Build history of the part. All positions in model axes, mm. A direction names the side the tool comes from. Round coordinates to 2 decimals unless told otherwise and drop trailing zeros. Order: outer loops, then holes, each group sorted by start corner. A loop starts at its lowest first (then second) coordinate and runs counter-clockwise, first axis right, second up. Notation, with made-up numbers: (49, 71.25) -> (100, 71.25) arc R5 ccw to (100, 78.25) -> close; hole circle Ø10 at (69, 1). An arc over 180 degrees is marked (long way). Write item = value, one per line.
from build123d import *

# Parameters (mm, degrees)
FILLET_1_R      = 0.3
FILLET_2_R      = 0.3
SKETCH_2_W      = 0.5
SKETCH_2_H      = 0.4
EXTRUDE_1_DEPTH = 5
SKETCH_3_W      = 0.7
SKETCH_3_H      = 0.6
EXTRUDE_2_DEPTH = 1.5
SKETCH_5_W      = 0.5
SKETCH_5_H      = 0.4
EXTRUDE_3_DEPTH = 9.5
SWEEP_START     = -1.52
SWEEP_2_DEPTH   = 0.5
SKETCH_7_262_W  = 0.5
SKETCH_7_262_H  = 0.4


# Read off the part's stored shape, not the designer's step: По траектории2
with BuildPart() as part:
    # Эскиз1 → Повернуть2 (revolve)
    with BuildSketch(Plane(origin=(0, 0, 0), x_dir=(0, 0, -1), z_dir=(1, 0, 0))):
        with BuildLine():
            Line((0, 0), (-2, 0))
            Line((-2, 0), (-2, 1))
            Line((-2, 1), (-1.5, 1))
            Line((-1.5, 1), (-1.5, 4))
            ThreePointArc((-1.5, 4), (-1.07971355, 5.07971355), (0, 5.5))
            Line((0, 5.5), (0, 0))
        make_face()
    revolve(axis=Axis((0, 5.5, 0), (0, -1, 0)))

    # Скругление1
    fillet_1_edges = [part.edges().sort_by_distance(p)[0] for p in [
        (0, 1, -2),
    ]]
    fillet(fillet_1_edges, radius=FILLET_1_R)

    # Скругление2
    fillet_2_edges = [part.edges().sort_by_distance(p)[0] for p in [
        (0, 1, -1.5),
    ]]
    fillet(fillet_2_edges, radius=FILLET_2_R)

    # Эскиз2 → Вытянуть1 (add)
    with BuildSketch(Plane.XZ):
        with Locations((-1.27, 0)):
            Rectangle(SKETCH_2_W, SKETCH_2_H)
        with Locations((1.27, 0)):
            Rectangle(SKETCH_2_W, SKETCH_2_H)
    extrude(amount=EXTRUDE_1_DEPTH)

    # Эскиз3 → Вытянуть2 (add)
    with BuildSketch(Plane.XZ.offset(5)):
        with Locations((-1.27, 0)):
            Rectangle(SKETCH_3_W, SKETCH_3_H)
        with Locations((1.27, 0)):
            Rectangle(SKETCH_3_W, SKETCH_3_H)
    extrude(amount=EXTRUDE_2_DEPTH)

    # Эскиз5 → Вытянуть3 (add)
    with BuildSketch(Plane.XZ.offset(6.5)):
        with Locations((-1.27, 0)):
            Rectangle(SKETCH_5_W, SKETCH_5_H)
        with Locations((1.27, 0)):
            Rectangle(SKETCH_5_W, SKETCH_5_H)
    extrude(amount=EXTRUDE_3_DEPTH)

    # По траектории2 outline → По траектории2 (add)
    with BuildSketch(Plane.YZ.offset(SWEEP_START)):
        with BuildLine():
            Line((-17.2, -3), (-16.8, -3))
            Line((-16.8, -3), (-16.8, -0.5))
            ThreePointArc((-16.8, -0.5), (-16.712132034, -0.287867966), (-16.5, -0.2))
            Line((-16.5, -0.2), (-16, -0.2))
            Line((-16, -0.2), (-16, 0.2))
            Line((-16, 0.2), (-16.5, 0.2))
            ThreePointArc((-16.5, 0.2), (-16.994974747, -0.005025253), (-17.2, -0.5))
            Line((-17.2, -0.5), (-17.2, -3))
        make_face()
    extrude(amount=SWEEP_2_DEPTH)

    # По траектории11: sweep along a curve in space
    with BuildLine() as sweep_11_path:
        Line((-1.27, -16, 0), (-1.27, -16.5, 0))
        ThreePointArc((-1.27, -16.5, 0), (-1.27, -16.853553391, -0.146446609), (-1.27, -17, -0.5))
        Line((-1.27, -17, -0.5), (-1.27, -17, -3))
    # Эскиз7<262> → По траектории11 (sweep)
    with BuildSketch(Plane.XZ.offset(16)):
        with Locations((-1.27, 0)):
            Rectangle(SKETCH_7_262_W, SKETCH_7_262_H)
        with Locations((1.27, 0)):
            Rectangle(SKETCH_7_262_W, SKETCH_7_262_H)
    sweep(path=sweep_11_path.line)


solid = part.part
Q1. Cut at A-A, the plane y = -6. List the corners of the cut face in (x, z).
Check values:
outline = (-1.62, -0.3) -> (-0.92, -0.3) -> (-0.92, 0.3) -> (-1.62, 0.3) -> close; (0.92, -0.3) -> (1.62, -0.3) -> (1.62, 0.3) -> (0.92, 0.3) -> close
Q2. Probe probe 1 along Y at (x, z) = (1.05, -2.15); probe 2 along Y at (x, z) = (0.95, -1.65); probe 3 along Z at (x, y) = (-1.2, -7). List the from-to ranges inside material, lowest first.
Check values:
probe_1 = -17.2 to -16.8
probe_2 = 0 to 0.92
probe_3 = -0.2 to 0.2
Q3. Cut at D-D, the plane y = 2. List the corners of the cut face in (x, z), and give its area (3 significant figures).
Check values:
outline = circle Ø3 at (0, 0)
area = 7.07 mm²
Q4. Cut at B-B, the plane y = -12.25. List the corners of the cut face in (x, z).
Check values:
outline = (-1.52, -0.2) -> (-1.02, -0.2) -> (-1.02, 0.2) -> (-1.52, 0.2) -> close; (1.02, -0.2) -> (1.52, -0.2) -> (1.52, 0.2) -> (1.02, 0.2) -> close
Q5. Flat gauge pins, fed straight in: pin 1 (0.8 mm diameter, centred on x = -1.5, y = -6, fed in from +Z); pin 2 (0.7 mm diameter, centred on x = 1.5, z = 0, fed in from +Y); pin 3 (1 mm diameter, centred on y = -4.5, z = -0.5, fed in from +X). Where does each tip first touch, or does it go through?
Check values:
pin_1 = 0.3
pin_2 = 5
pin_3 = 1.52
Q6. Which spindle directions (+Z, -Z, +X, -X, +Y, -Y) get a long thin tool onto all of the face, cutting with end or side? Do faces 1 (the face through (-1.02, -13, 0)), 2 (the face through (1.952, 0.355, -0.434)), 3 (the face through (1.52, -13, 0)). Say none if no direction does.
Check values:
face_1 = +Z, -Z, -Y
face_2 = +Y
face_3 = +Z, -Z, +X, -Y
Q7. Cut at C-C, the plane z = -1.3. Give the number of separate pieces and of enclosed holes in the cut face, and give its area (3 significant figures).
Check values:
separate_pieces = 3
enclosed_holes = 0
area = 8.90 mm²
